The model under review builds one solid part; all positions refer to its coordinate system, in mm. A direction names the side the tool comes from. Coordinates: 2 decimals unless noted, no trailing zeros. Loops run counter-clockwise (first coordinate to the right, second up) from the corner with the lowest first, then second, coordinate; pieces in that order, holes last. Notation, with made-up numbers: M 82,45.25 L 122,45.25 A4 cw 122,49.25 Z; hole C 1,42 d6. An arc over 180 degrees is marked long. Write item = value, one per line. Start each with the question number.
Q1. Wall thickness on probe 1 along Z at (x, y) = (-0.5, -4.75); probe 2 along Z at (x, y) = (-5.5, -0.5); probe 3 along X at (y, z) = (-0.25, 37): over which ranges is each line inside the solid? List them lowest first.
Q2. We need section A-A on y = 0. Give the boundary of the cut face in (x, z).
Q3. Mouldability with a two-part tool opening along Z and no side actions: class faces 3 (the face through (4, 4, 0)), 4 (the face through (-1.08, -4.88, 13.31)), 5 (the face through (2.5, 3.92, 27.54)) as released by +Z, released by -Z, zero draft, split by the parting line, or undercut.
Q4. We need section C-C on z = -7. Give the boundary of the cut face in (x, y).
Q5. Clearance check with a flat-ended pin moving along its axis: pin 1 Ø5 at (y, z) = (-4, -1) entering from -X. State where the tip first meets the part, or that it passes through.
Q6. For faces 1 (the face through (0, 0, -40)), 2 (the face through (5, 0, 35)), list the 3-axis set-ups (+Z, -Z, +X, -X, +Y, -Y) from which the entire face can be reached by the end or side of a thin tool; tool diameter is ignored.
Q7. We need section D-D on z = 33.5. Give the boundary of the cut face in (x, y).
from build123d import *

# Parameters (mm, degrees)
SKETCH_1_R      = 5
EXTRUDE_1_DEPTH = 27
SKETCH_2_R      = 6
EXTRUDE_2_DEPTH = 40
SKETCH_3_R      = 4.65
EXTRUDE_3_DEPTH = 1.1
SKETCH_4_R      = 5
EXTRUDE_4_DEPTH = 15


with BuildPart() as part:
    # 草图1 → 凸台-拉伸1 (new body)
    with BuildSketch(Plane.XY):
        Circle(SKETCH_1_R)
    extrude(amount=EXTRUDE_1_DEPTH)

    # 草图2 → 凸台-拉伸2 (add)
    with BuildSketch(Plane(origin=(0, 0, 0), x_dir=(-1, 0, 0), z_dir=(0, 0, -1))):
        Circle(SKETCH_2_R)
    extrude(amount=EXTRUDE_2_DEPTH)

    # 草图3 → 凸台-拉伸3 (add)
    with BuildSketch(Plane.XY.offset(27)):
        Circle(SKETCH_3_R)
    extrude(amount=EXTRUDE_3_DEPTH)

    # 草图4 → 凸台-拉伸4 (add)
    with BuildSketch(Plane.XY.offset(28.1)):
        with Locations(Location((0, 0, 0), (0, 0, 180))):
            Circle(SKETCH_4_R)
    extrude(amount=EXTRUDE_4_DEPTH)


solid = part.part
Returned:
q1.probe_1 = -40 to 27, 28.1 to 43.1
q1.probe_2 = -40 to 0
q1.probe_3 = -4.99 to 4.99
q2.outline = M -6,-40 L 6,-40 L 6,0 L 5,0 L 5,27 L 4.65,27 L 4.65,28.1 L 5,28.1 L 5,43.1 L -5,43.1 L -5,28.1 L -4.65,28.1 L -4.65,27 L -5,27 L -5,0 L -6,0 Z
q3.face_3 = released by +Z
q3.face_4 = zero draft
q3.face_5 = undercut
q4.outline = C 0,0 d12
q5.pin_1 = -5.81
q6.face_1 = -Z, +X, -X, +Y, -Y
q6.face_2 = +Z
q7.outline = C 0,0 d10
